Read the model definition and answer for the solid it produces. Units are mm, in the model's axes. Face numbers are marked on the shaded views. Coordinates: 2 decimals unless noted, no trailing zeros. Loops run counter-clockwise (first coordinate to the right, second up) from the corner with the lowest first, then second, coordinate; pieces in that order, holes last. Notation, with made-up numbers: (55.5, 20.25) -> (89.5, 20.25) arc R21 ccw to (89.5, 56.25) -> close; hole circle Ø3 at (-19.75, -9). An arc over 180 degrees is marked (long way). Answer as a JSON object with one key per item and string values. Group by question number.
Q1. The part is cut by section D-D on z = 2. Write down the section's boundary in (x, y).
Q2. Straight lines are drawn through the part: line 1 along Z through (x, y) = (1.4, -5.5); line 2 along Z through (x, y) = (3.9, -3.25); line 3 along Y through (x, z) = (3.6, 2.75). For each, find the intervals that lie inside material, in ascending order. Write a range as [from, to].
Q3. Determine the mould class of the marked faces 1, 2, 3 and 4 for opening direction Z: released by +Z, released by -Z, zero draft, split by the parting line, or undercut.
Q4. The part is cut by section A-A on y = 0. Write down the section's boundary in (x, z).
Q5. The part is cut by section B-B on z = 0. Write down the section's boundary in (x, y).
Q6. The part is cut by section C-C on x = 1.45. Write down the section's boundary in (y, z), and give its area (3 significant figures).
from build123d import *

# Parameters (mm, degrees)
SKETCH1_R           = 1.7272
SKETCH1_R_2         = 3.81
BOSS_EXTRUDE1_DEPTH = 4.826


with BuildPart() as part:
    # Sketch1 → Boss-Extrude1 (new body)
    with BuildSketch(Plane(origin=(0, 0, 0), x_dir=(0, 0, -1), z_dir=(1, 0, 0))):
        with BuildLine():
            Line((-7.5, 9.367496998), (-7.5, -9.367496998))
            ThreePointArc((-7.5, -9.367496998), (0, -12), (7.5, -9.367496998))
            Line((7.5, -9.367496998), (7.5, 9.367496998))
            ThreePointArc((7.5, 9.367496998), (0, 12), (-7.5, 9.367496998))
        make_face()
        with Locations((0, 7)):
            Circle(SKETCH1_R, mode=Mode.SUBTRACT)
        with Locations((0, -7)):
            Circle(SKETCH1_R, mode=Mode.SUBTRACT)
        Circle(SKETCH1_R_2, mode=Mode.SUBTRACT)
    extrude(amount=BOSS_EXTRUDE1_DEPTH)


solid = part.part
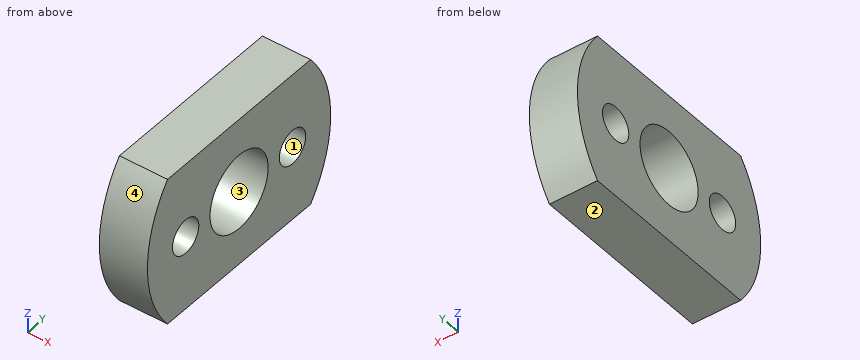
Final values:
{
 "1": {"outline": "(0, -11.83) -> (4.83, -11.83) -> (4.83, -3.24) -> (0, -3.24) -> close; (0, 3.24) -> (4.83, 3.24) -> (4.83, 11.83) -> (0, 11.83) -> close"},
 "2": {"line 1": "z = [-7.5, -0.86], [0.86, 7.5]", "line 2": "z = [-7.5, -1.99], [1.99, 7.5]", "line 3": "y = [-11.68, -2.64], [2.64, 11.68]"},
 "3": {"face 1": "undercut", "face 2": "released by -Z", "face 3": "undercut", "face 4": "split by the parting line"},
 "4": {"outline": "(0, -7.5) -> (4.83, -7.5) -> (4.83, -3.81) -> (0, -3.81) -> close; (0, 3.81) -> (4.83, 3.81) -> (4.83, 7.5) -> (0, 7.5) -> close"},
 "5": {"outline": "(0, -12) -> (4.83, -12) -> (4.83, -8.73) -> (0, -8.73) -> close; (0, -5.27) -> (4.83, -5.27) -> (4.83, -3.81) -> (0, -3.81) -> close; (0, 3.81) -> (4.83, 3.81) -> (4.83, 5.27) -> (0, 5.27) -> close; (0, 8.73) -> (4.83, 8.73) -> (4.83, 12) -> (0, 12) -> close"},
 "6": {"outline": "(-9.37, -7.5) -> (9.37, -7.5) arc R12 ccw to (9.37, 7.5) -> (-9.37, 7.5) arc R12 ccw to start; hole circle Ø3.45 at (-7, 0); hole circle Ø7.62 at (0, 0); hole circle Ø3.45 at (7, 0)", "area": "271 mm2"}
}
